Geometry: final body of the model. Coordinates: model frame, mm. Face numbers are marked on the shaded views. A direction names the side the tool comes from. Coordinates: 2 decimals unless noted, no trailing zeros. Loops run counter-clockwise (first coordinate to the right, second up) from the corner with the lowest first, then second, coordinate; pieces in that order, holes last. Notation, with made-up numbers: (-39, -10) - (-32, -10) arc R18 cw to (-32, -4) - close; hole circle Ø3 at (67, 0.5). An arc over 180 degrees is marked (long way). Return JSON: item names as keys, results as strings.
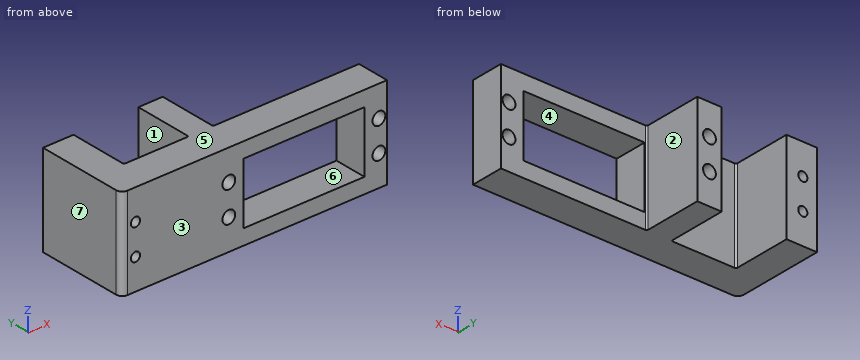
from build123d import *

# Parameters (mm, degrees)
SKETCH1_W           = 77.1
SKETCH1_H           = 30
SKETCH1_W_2         = 39.7
SKETCH1_H_2         = 20
BOSS_EXTRUDE1_DEPTH = 10.7
SKETCH4_W           = 30
SKETCH4_H           = 30
BOSS_EXTRUDE3_DEPTH = 10
CUT_EXTRUDE2_REACH  = 62.083
SKETCH6_R           = 2.1
FILLET5_R           = 2
FILLET6_R           = 0.5
CUT_EXTRUDE3_REACH  = 62.083
SKETCH7_R           = 1.5
SKETCH9_W           = 8
SKETCH9_H           = 30
SKETCH9_R           = 2.1
BOSS_EXTRUDE4_DEPTH = 19.3
FILLET7_R           = 0.5


with BuildPart() as part:
    # Sketch1 → Boss-Extrude1 (new body)
    with BuildSketch(Plane(origin=(0, 0, 0), x_dir=(1, 0, 0), z_dir=(0, 1, 0))):
        with Locations((11.3, 0)):
            Rectangle(SKETCH1_W, SKETCH1_H)
        with Locations((22.6, 0)):
            Rectangle(SKETCH1_W_2, SKETCH1_H_2, mode=Mode.SUBTRACT)
    extrude(amount=BOSS_EXTRUDE1_DEPTH)

    # Sketch4 → Boss-Extrude3 (add)
    with BuildSketch(Plane.ZY.offset(27.25)):
        with Locations((0, 15)):
            Rectangle(SKETCH4_W, SKETCH4_H)
    extrude(amount=BOSS_EXTRUDE3_DEPTH)

    # Sketch6 → Cut-Extrude2 (cut, up to next)
    with BuildSketch(Plane(origin=(0, 0, 0), x_dir=(-1, 0, 0), z_dir=(0, -1, 0)), mode=Mode.PRIVATE) as cut_extrude2_sk1:
        with Locations(Location((2, 5, 0), (0, 0, 90))):
            Circle(SKETCH6_R)
    cut_extrude2_tool1 = extrude(cut_extrude2_sk1.sketch, amount=-CUT_EXTRUDE2_REACH, mode=Mode.PRIVATE) & part.part
    # Sketch6 → Cut-Extrude2 (cut, up to next)
    with BuildSketch(Plane(origin=(0, 0, 0), x_dir=(-1, 0, 0), z_dir=(0, -1, 0)), mode=Mode.PRIVATE) as cut_extrude2_sk2:
        with Locations(Location((2, -5, 0), (0, 0, 90))):
            Circle(SKETCH6_R)
    cut_extrude2_tool2 = extrude(cut_extrude2_sk2.sketch, amount=-CUT_EXTRUDE2_REACH, mode=Mode.PRIVATE) & part.part
    # Sketch6 → Cut-Extrude2 (cut, up to next)
    with BuildSketch(Plane(origin=(0, 0, 0), x_dir=(-1, 0, 0), z_dir=(0, -1, 0)), mode=Mode.PRIVATE) as cut_extrude2_sk3:
        with Locations(Location((-47.2, 5, 0), (0, 0, 90))):
            Circle(SKETCH6_R)
    cut_extrude2_tool3 = extrude(cut_extrude2_sk3.sketch, amount=-CUT_EXTRUDE2_REACH, mode=Mode.PRIVATE) & part.part
    # Sketch6 → Cut-Extrude2 (cut, up to next)
    with BuildSketch(Plane(origin=(0, 0, 0), x_dir=(-1, 0, 0), z_dir=(0, -1, 0)), mode=Mode.PRIVATE) as cut_extrude2_sk4:
        with Locations(Location((-47.2, -5, 0), (0, 0, 90))):
            Circle(SKETCH6_R)
    cut_extrude2_tool4 = extrude(cut_extrude2_sk4.sketch, amount=-CUT_EXTRUDE2_REACH, mode=Mode.PRIVATE) & part.part
    add(cut_extrude2_tool1.solids().sort_by_distance((-2, 0, -5))[0], mode=Mode.SUBTRACT)
    add(cut_extrude2_tool2.solids().sort_by_distance((-2, 0, 5))[0], mode=Mode.SUBTRACT)
    add(cut_extrude2_tool3.solids().sort_by_distance((47.2, 0, -5))[0], mode=Mode.SUBTRACT)
    add(cut_extrude2_tool4.solids().sort_by_distance((47.2, 0, 5))[0], mode=Mode.SUBTRACT)

    # Fillet5
    fillet5_edges = [part.edges().sort_by_distance(p)[0] for p in [
        (-37.25, 0, 0),
    ]]
    fillet(fillet5_edges, radius=FILLET5_R)

    # Fillet6
    fillet6_edges = [part.edges().sort_by_distance(p)[0] for p in [
        (-27.25, 10.7, 0),
    ]]
    fillet(fillet6_edges, radius=FILLET6_R)

    # Sketch7 → Cut-Extrude3 (cut, up to next)
    with BuildSketch(Plane(origin=(0, 0, 0), x_dir=(-1, 0, 0), z_dir=(0, -1, 0)), mode=Mode.PRIVATE) as cut_extrude3_sk1:
        with Locations(Location((32.6, -5, 0), (0, 0, 90))):
            Circle(SKETCH7_R)
    cut_extrude3_tool1 = extrude(cut_extrude3_sk1.sketch, amount=-CUT_EXTRUDE3_REACH, mode=Mode.PRIVATE) & part.part
    # Sketch7 → Cut-Extrude3 (cut, up to next)
    with BuildSketch(Plane(origin=(0, 0, 0), x_dir=(-1, 0, 0), z_dir=(0, -1, 0)), mode=Mode.PRIVATE) as cut_extrude3_sk2:
        with Locations(Location((32.6, 5, 0), (0, 0, 90))):
            Circle(SKETCH7_R)
    cut_extrude3_tool2 = extrude(cut_extrude3_sk2.sketch, amount=-CUT_EXTRUDE3_REACH, mode=Mode.PRIVATE) & part.part
    add(cut_extrude3_tool1.solids().sort_by_distance((-32.6, 0, 5))[0], mode=Mode.SUBTRACT)
    add(cut_extrude3_tool2.solids().sort_by_distance((-32.6, 0, -5))[0], mode=Mode.SUBTRACT)

    # Sketch9 → Boss-Extrude4 (add)
    with BuildSketch(Plane(origin=(0, 10.7, 0), x_dir=(1, 0, 0), z_dir=(0, 1, 0))):
        with Locations((-2, 0)):
            Rectangle(SKETCH9_W, SKETCH9_H)
        with Locations(Location((-2, 5, 0), (0, 0, 90))):
            Circle(SKETCH9_R, mode=Mode.SUBTRACT)
        with Locations(Location((-2, -5, 0), (0, 0, 90))):
            Circle(SKETCH9_R, mode=Mode.SUBTRACT)
    extrude(amount=BOSS_EXTRUDE4_DEPTH)

    # Fillet7
    fillet7_edges = [part.edges().sort_by_distance(p)[0] for p in [
        (-6, 10.7, 0),
        (2, 10.7, 0),
    ]]
    fillet(fillet7_edges, radius=FILLET7_R)


solid = part.part
Item 1: First-contact query: pin 1 Ø8 at (y, z) = (18, -10.5) entering from +X; pin 2 Ø6.5 at (x, z) = (47.2, 5) entering from +Y. Flat tips, straight axial feed; report the tip coordinate or a pass-through.
Worked out:
{"pin 1": "x = 2", "pin 2": "y = 10.7"}
Item 2: Section query C-C, the plane z = 2. Return loops of the section in (x, y), and give its area (3 significant figures).
Worked out:
{"outline": "(-37.25, 2) arc R2 ccw to (-35.25, 0) - (2.75, 0) - (2.75, 10.7) - (2.5, 10.7) arc R0.5 cw to (2, 11.2) - (2, 30) - (-6, 30) - (-6, 11.2) arc R0.5 cw to (-6.5, 10.7) - (-26.75, 10.7) arc R0.5 cw to (-27.25, 11.2) - (-27.25, 30) - (-37.25, 30) - close; (42.45, 0) - (49.85, 0) - (49.85, 10.7) - (42.45, 10.7) - close", "area": "854 mm^2"}
Item 3: Mould query, pull axis Z, two halves, no side actions, for the marked faces 5, 6 and 7. Classes: +Z half, -Z half, draft (parallel to the pull), parting line (faces both ways), or undercut.
Worked out:
{"face 5": "+Z half", "face 6": "undercut", "face 7": "draft"}
Item 4: Reachability of the marked faces 1, 2, 3 and 4 from +Z, -Z, +X, -X, +Y, -Y: full face, straight path, thin tool, end or side. Return the list, or none.
Worked out:
{"face 1": "+Z, -Z, +Y", "face 2": "+Z, -Z, +X, +Y", "face 3": "+Z, -Z, +X, -X, -Y", "face 4": "+Y, -Y"}
Item 5: Section query D-D, the plane y = 3.75. Return loops of the section in (x, z).
Worked out:
{"outline": "(-37.25, -15) - (49.85, -15) - (49.85, 15) - (-37.25, 15) - close; hole circle Ø3 at (-32.6, -5); hole circle Ø3 at (-32.6, 5); hole circle Ø4.2 at (-2, -5); hole circle Ø4.2 at (-2, 5); hole (2.75, -10) - (42.45, -10) - (42.45, 10) - (2.75, 10) - close; hole circle Ø4.2 at (47.2, -5); hole circle Ø4.2 at (47.2, 5)"}
Item 6: Ray query, probe 1 along Z at (x, y) = (-2, 17); probe 2 along X at (y, z) = (6.5, 5); probe 3 along X at (y, z) = (25.75, -13.5). Return the intervals inside material, ascending. Write a range as from..to.
Worked out:
{"probe 1": "-15..-7.1, -2.9..2.9, 7.1..15", "probe 2": "-37.25..-34.1, -31.1..-4.1, 0.1..2.75, 42.45..45.1, 49.3..49.85", "probe 3": "-37.25..-27.25, -6..2"}
Item 7: Section query B-B, the plane x = -2. Return loops of the section in (y, z), and give its area (3 significant figures).
Worked out:
{"outline": "(0, -15) - (30, -15) - (30, -7.1) - (0, -7.1) - close; (0, -2.9) - (30, -2.9) - (30, 2.9) - (0, 2.9) - close; (0, 7.1) - (30, 7.1) - (30, 15) - (0, 15) - close", "area": "648 mm^2"}
Item 8: Section query A-A, the plane y = 12. Return loops of the section in (x, z), and give its area (3 significant figures).
Worked out:
{"outline": "(-37.25, -15) - (-27.25, -15) - (-27.25, 15) - (-37.25, 15) - close; (-6, -15) - (2, -15) - (2, 15) - (-6, 15) - close; hole circle Ø3 at (-32.6, -5); hole circle Ø3 at (-32.6, 5); hole circle Ø4.2 at (-2, -5); hole circle Ø4.2 at (-2, 5)", "area": "498 mm^2"}
